from build123d import *

# Parameters (mm, degrees)
ESQUISSE1_W             = 3
ESQUISSE1_H             = 3
BOSS_EXTRU_1_DEPTH      = 95
ESQUISSE2_R             = 2.5
BOSS_EXTRU_2_DEPTH      = 1
ESQUISSE3_W             = 3
ESQUISSE3_H             = 3
ENL_V_MAT_EXTRU_1_DEPTH = 17


with BuildPart() as part:
    # Esquisse1 → Boss.-Extru.1 (new body)
    with BuildSketch(Plane(origin=(0, 0, 0), x_dir=(1, 0, 0), z_dir=(0, 1, 0))):
        Rectangle(ESQUISSE1_W, ESQUISSE1_H)
    extrude(amount=BOSS_EXTRU_1_DEPTH)

    # Esquisse2 → Boss.-Extru.2 (add)
    with BuildSketch(Plane.XZ):
        with Locations(Location((0, 0, 0), (0, 0, 270))):
            Circle(ESQUISSE2_R)
    extrude(amount=BOSS_EXTRU_2_DEPTH)

    # Esquisse3 → Enlèv. mat.-Extru.1 (cut)
    with BuildSketch(Plane(origin=(0, 95, 0), x_dir=(1, 0, 0), z_dir=(0, 1, 0))):
        Rectangle(ESQUISSE3_W, ESQUISSE3_H)
    extrude(amount=-ENL_V_MAT_EXTRU_1_DEPTH, mode=Mode.SUBTRACT)


solid = part.part
Source: CAD feature listing. Evaluate the final solid. Frame: model axes, mm. A direction names the side the tool comes from. Give positions to 0.01 mm unless a question says otherwise; leave off trailing zeros. Order: outer loops, then holes, each group sorted by start corner. A loop starts at its lowest first (then second) coordinate and runs counter-clockwise, first axis right, second up. Notation, with made-up numbers: (65.5, 70) -> (85.5, 70) arc R22 ccw to (85.5, 109) -> close; hole circle Ø8 at (-1, 8.5). An arc over 180 degrees is marked (long way). Use a Markdown table: item, result.
1) Section query C-C, the plane y = 61.5. Return the cut outline in (x, z), then the cut area to 3 significant figures.
Answer list:
| item | result |
|---|---|
| outline | (-1.5, -1.5) -> (1.5, -1.5) -> (1.5, 1.5) -> (-1.5, 1.5) -> close |
| area | 9.00 mm² |
2) Ray query, line 1 along X through (y, z) = (67, -1.05); line 2 along Y through (x, z) = (2, 1.45). Return the intervals inside material, ascending. Write a range as [from, to].
Answer list:
| item | result |
|---|---|
| line 1 | [-1.5, 1.5] |
| line 2 | [-1, 0] |
3) Section query A-A, the plane x = 0. Return the cut outline in (y, z).
Answer list:
| item | result |
|---|---|
| outline | (-1, -2.5) -> (0, -2.5) -> (0, -1.5) -> (78, -1.5) -> (78, 1.5) -> (0, 1.5) -> (0, 2.5) -> (-1, 2.5) -> close |
4) Contact query for flat-ended pins moving along their axis: P1, Ø2, axis at y = 59, z = 0.5, coming from the +X side; P2, Ø1.5, axis at x = -0.5, y = 40, coming from the -Z side; P3, Ø1, axis at x = -1, y = 37.5, coming from the +Z side. Output: stop coordinate, or through.
Answer list:
| item | result |
|---|---|
| P1 | x = 1.5 |
| P2 | z = -1.5 |
| P3 | z = 1.5 |
5) Section query B-B, the plane z = 0. Return the cut outline in (x, y), then the cut area to 3 significant figures.
Answer list:
| item | result |
|---|---|
| outline | (-2.5, -1) -> (2.5, -1) -> (2.5, 0) -> (1.5, 0) -> (1.5, 78) -> (-1.5, 78) -> (-1.5, 0) -> (-2.5, 0) -> close |
| area | 239 mm² |
6) Reachability of faces 1 (the flat face through (-1.5, 38, 0)), 2 (the flat face through (0, 78, 0)), 3 (the flat face through (0, 38, 1.5)), 4 (the flat face through (0, 38, -1.5)), 5 (the flat face through (1.5, 38, 0)) from +Z, -Z, +X, -X, +Y, -Y: full face, straight path, thin tool, end or side. Return the list, or none.
Answer list:
| item | result |
|---|---|
| face 1 | +Z, -Z, -X, +Y |
| face 2 | +Z, -Z, +X, -X, +Y |
| face 3 | +Z, +X, -X, +Y |
| face 4 | -Z, +X, -X, +Y |
| face 5 | +Z, -Z, +X, +Y |
